from build123d import *

# Parameters (mm, degrees)
F0_R     = 2.5
F1_DEPTH = 3.175
F2_W     = 12.7
F2_H     = 3.175
F2_W_2   = 74.1
F3_DEPTH = 9.525
F4_W     = 12.7
F4_H     = 3.175
F5_DEPTH = 3.175
F6_W     = 74.1
F6_H     = 3.175
F7_DEPTH = 3.175
F8_R     = 3.17499


# Not quite as in the source:
# - a fillet or chamfer is up to 0.001 mm smaller than in the source, because OpenCascade refuses the exact size


with BuildPart() as f1:
    # F0 (on Front) → F1 (new body)
    with BuildSketch(Plane.XZ):
        Polygon((49.75, -15.875), (49.75, 15.875), (-49.75, 15.875), (-49.75, -15.875), (-37.05, -15.875), (-37.05, 3.175), (37.05, 3.175), (37.05, -15.875), align=None)
        with Locations((-43, 9.125)):
            Circle(F0_R, mode=Mode.SUBTRACT)
        with Locations((43, 9.125)):
            Circle(F0_R, mode=Mode.SUBTRACT)
    extrude(amount=F1_DEPTH)

    # F2 (on face) → F3 (join)
    with BuildSketch(Plane.XZ.offset(3.175)):
        with Locations((-43.4, -14.2875)):
            Rectangle(F2_W, F2_H)
        with Locations((43.4, -14.2875)):
            Rectangle(F2_W, F2_H)
        with Locations((0, 14.2875)):
            Rectangle(F2_W_2, F2_H)
    extrude(amount=F3_DEPTH)

    # F4 (on face) → F5 (join)
    with BuildSketch(Plane.XY.offset(-12.7)):
        with Locations((-43.4, -11.1125)):
            Rectangle(F4_W, F4_H)
        with Locations((43.4, -11.1125)):
            Rectangle(F4_W, F4_H)
    extrude(amount=F5_DEPTH)

    # F6 (on face) → F7 (join)
    with BuildSketch(Plane(origin=(0, 0, 12.7), x_dir=(1, 0, 0), z_dir=(0, 0, -1))):
        with Locations((0, 11.1125)):
            Rectangle(F6_W, F6_H)
    extrude(amount=F7_DEPTH)

    # F8 (radius 3.175 in the source; OpenCascade refuses exactly that, so slightly less here)
    f8_edges = [f1.edges().sort_by_distance(p)[0] for p in [
        (-49.75, -1.5875, 15.875),
        (-49.75, -6.35, -15.875),
        (-37.05, -6.35, -15.875),
        (49.75, -6.35, -15.875),
        (37.05, -6.35, -15.875),
        (49.75, -1.5875, 15.875),
        (37.05, -1.5875, 3.175),
        (-37.05, -1.5875, 3.175),
        (-49.75, -11.1125, -9.525),
        (-37.05, -11.1125, -9.525),
        (49.75, -11.1125, -9.525),
        (37.05, -11.1125, -9.525),
        (-37.05, -7.9375, 15.875),
        (-37.05, -11.1125, 9.525),
        (37.05, -7.9375, 15.875),
        (37.05, -11.1125, 9.525),
    ]]
    fillet(f8_edges, radius=F8_R)


solid = f1.part
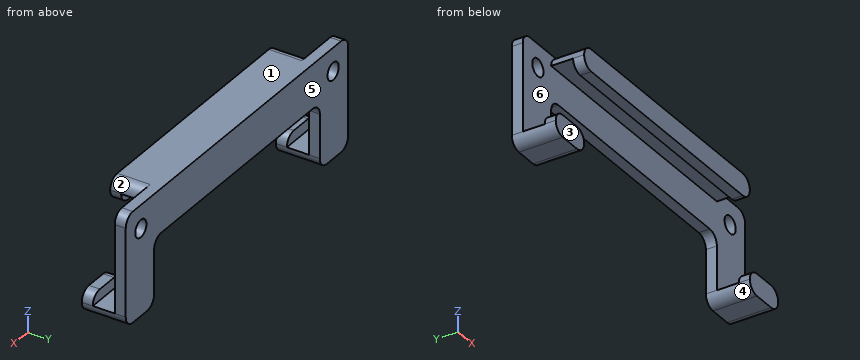
Verification items for the finished model (mm, model axes). Face numbers are marked on the shaded views. A direction names the side the tool comes from. Round coordinates to 2 decimals unless told otherwise and drop trailing zeros. Loops run counter-clockwise (first coordinate to the right, second up) from the corner with the lowest first, then second, coordinate; pieces in that order, holes last. Notation, with made-up numbers: M -9,32.5 L 10,32.5 A16 cw 10,36.5 Z; hole C -32,2.5 d2. An arc over 180 degrees is marked long. Write each question's results on one line, items separated by ' | '.
1) Mould release check, pull along Y, two halves, no side actions. Record for the marked faces 3, 4, 5 and 6: released by +Y, released by -Y, zero draft, split by the parting line, or undercut.
Checks:
face 3: released by -Y | face 4: zero draft | face 5: released by +Y | face 6: undercut
2) Section check D-D on x = 2. Record the boundary of the cut face in (y, z) (3 decimals).
Checks:
outline: M -12.7,9.525 L -9.525,9.525 L -9.525,12.7 L -3.175,12.7 L -3.175,3.175 L 0,3.175 L 0,15.875 L -12.7,15.875 Z
3) Section check A-A on z = -1.5. Record the boundary of the cut face in (x, y) (3 decimals).
Checks:
outline: M -49.75,-3.175 L -37.05,-3.175 L -37.05,0 L -49.75,0 Z; M 37.05,-3.175 L 49.75,-3.175 L 49.75,0 L 37.05,0 Z
4) Section check C-C on y = -6.75. State how many separate pieces and enclosed holes the cut face has, then the cut area to 3 significant figures.
Checks:
separate pieces: 3 | enclosed holes: 0 | area: 303 mm2
5) Scan lines: L1, parallel to Z at x = -43, y = -2.45 (3 decimals); L2, parallel to X at y = -2.75, z = -8; L3, parallel to Y at x = -2.5, z = 11 (3 decimals). Record each from-to range of solid material in increasing order. Write a range as from..to.
Checks:
L1: z = -15.875..6.625, 11.625..15.875 | L2: x = -49.75..-37.05, 37.05..49.75 | L3: y = -12.7..-9.525, -3.175..0
6) Access from +Z, -Z, +X, -X, +Y, -Y to the whole of each face (thin tool, end or side, straight path). Record for the marked faces 1 and 2.
Checks:
face 1: +Z, +X, -X, +Y, -Y | face 2: +Z, +X, -Y
7) Section check B-B on x = 43. Record the boundary of the cut face in (y, z) (3 decimals).
Checks:
outline: M -12.7,-15.875 L 0,-15.875 L 0,6.625 L -3.175,6.625 L -3.175,-12.7 L -9.525,-12.7 L -9.525,-9.525 L -12.7,-9.525 Z; M -3.175,11.625 L 0,11.625 L 0,15.875 L -3.175,15.875 Z
8) Gauge pin test, flat ends, axial feed: P1, Ø2, axis at y = -8, z = 11, coming from the -X side; P2, Ø1, axis at x = 11, y = -11, coming from the -Z side (3 decimals); P3, Ø1.6, axis at x = 42, y = -11, coming from the +Z side (3 decimals); P4, Ø1.9, axis at x = 8, y = -7.5, coming from the -Z side. Record the tip position at first contact, or that the pin passes through.
Checks:
P1: passes through | P2: stops at z = 9.525 | P3: stops at z = -9.525 | P4: stops at z = 12.7
